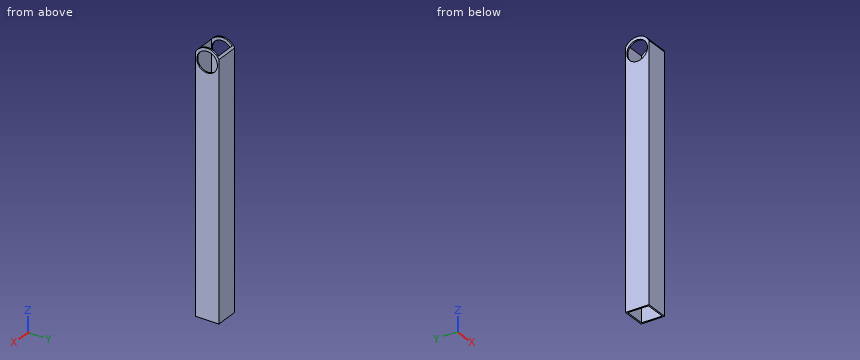
from build123d import *

# Parameters (mm, degrees)
SKETCH1_W           = 25.4
SKETCH1_H           = 25.4
SKETCH1_W_2         = 22.225
SKETCH1_H_2         = 22.225
EXTRUDE_THIN1_DEPTH = 142.24
SKETCH2_R           = 11.1125
CUT_EXTRUDE1_DEPTH  = 146.047121998
CUT_EXTRUDE2_DEPTH  = 146.047121998


with BuildPart() as part:
    # Sketch1 → Extrude-Thin1 (new, symmetric)
    with BuildSketch(Plane.XY):
        Rectangle(SKETCH1_W, SKETCH1_H)
        Rectangle(SKETCH1_W_2, SKETCH1_H_2, mode=Mode.SUBTRACT)
    extrude(amount=EXTRUDE_THIN1_DEPTH, both=True)

    # Sketch2 → Cut-Extrude1 (cut, through all)
    with BuildSketch(Plane(origin=(12.7, 0, 0), x_dir=(0, 0, -1), z_dir=(1, 0, 0))):
        with Locations((-123.19, 0)):
            Circle(SKETCH2_R)
    extrude(amount=-CUT_EXTRUDE1_DEPTH, mode=Mode.SUBTRACT)

    # Sketch3 → Cut-Extrude2 (cut, through all)
    with BuildSketch(Plane(origin=(12.7, 0, 0), x_dir=(0, 0, -1), z_dir=(1, 0, 0))):
        with BuildLine():
            Line((-123.19, 14.2875), (-142.24, 14.2875))
            Line((-142.24, 14.2875), (-142.24, -12.7))
            Line((-142.24, -12.7), (-129.735430181, -12.7))
            ThreePointArc((-129.735430181, -12.7), (-137.0749542, 3.367596045), (-123.19, 14.2875))
        make_face()
    extrude(amount=-CUT_EXTRUDE2_DEPTH, mode=Mode.SUBTRACT)


solid = part.part
Source: CAD feature listing. Evaluate the final solid. Frame: model axes, mm. Coordinates: 2 decimals unless noted, no trailing zeros. Order: outer loops, then holes, each group sorted by start corner. A loop starts at its lowest first (then second) coordinate and runs counter-clockwise, first axis right, second up.
Item 1: Cut plane B-B (y = 0). Return loops of the section in (x, z), plus the area to 3 significant figures.
Output values:
outline: (-12.7, -142.24) - (-11.11, -142.24) - (-11.11, 112.08) - (-12.7, 112.08) - close; (-12.7, 134.3) - (-11.11, 134.3) - (-11.11, 137.48) - (-12.7, 137.48) - close; (11.11, -142.24) - (12.7, -142.24) - (12.7, 112.08) - (11.11, 112.08) - close; (11.11, 134.3) - (12.7, 134.3) - (12.7, 137.48) - (11.11, 137.48) - close
area: 818 mm2
Item 2: Cut plane A-A (x = -2.75). Return loops of the section in (y, z) (1 decimal), plus the area to 3 significant figures.
Output values:
outline: (-12.7, -142.2) - (-11.1, -142.2) - (-11.1, 132.2) arc R14.3 ccw to (-12.7, 129.7) - close; (11.1, -142.2) - (12.7, -142.2) - (12.7, 129.7) arc R14.3 ccw to (11.1, 132.2) - close
area: 868 mm2
Item 3: Cut plane C-C (z = -78.5). Return loops of the section in (x, y).
Output values:
outline: (-12.7, -12.7) - (12.7, -12.7) - (12.7, 12.7) - (-12.7, 12.7) - close; hole (-11.11, -11.11) - (11.11, -11.11) - (11.11, 11.11) - (-11.11, 11.11) - close
Item 4: Material intervals for line 1 (Z direction, x = -11.95, y = 0); line 2 (X direction, y = 3.5, z = -55.5), sorted ascending.
Output values:
line 1: z = -142.24 to 112.08, 134.3 to 137.48
line 2: x = -12.7 to -11.11, 11.11 to 12.7
